from build123d import *

# Parameters (mm, degrees)
SKETCH1_R                   = 7.9375
BOSS_EXTRUDE1_DEPTH         = 9.525
SKETCH2_R                   = 4.7625
BOSS_EXTRUDE2_DEPTH         = 3.175
F_1_4_0_25_DIAMETER_HOLE1_D = 6.35
F_10_32_TAPPED_HOLE1_REACH  = 23.825
F_10_32_TAPPED_HOLE1_BORE_R = 2.0193


with BuildPart() as part:
    # Sketch1 → Boss-Extrude1 (new body)
    with BuildSketch(Plane(origin=(0, 0, 0), x_dir=(1, 0, 0), z_dir=(0, 1, 0))):
        with Locations(Location((0, 0, 0), (0, 0, 90))):
            Circle(SKETCH1_R)
    extrude(amount=BOSS_EXTRUDE1_DEPTH)

    # Sketch2 → Boss-Extrude2 (add)
    with BuildSketch(Plane(origin=(0, 9.525, 0), x_dir=(1, 0, 0), z_dir=(0, 1, 0))):
        with Locations(Location((0, 0, 0), (0, 0, 270))):
            Circle(SKETCH2_R)
    extrude(amount=BOSS_EXTRUDE2_DEPTH)

    # 1/4 (0.25) Diameter Hole1 (through all)
    with Locations(Plane(origin=(0, 0, 0), x_dir=(-1, 0, 0), z_dir=(0, -1, 0))):
        with Locations((0, 0)):
            Hole(F_1_4_0_25_DIAMETER_HOLE1_D / 2)

    # #10-32 Tapped Hole1 bore → #10-32 Tapped Hole1 (cut, up to next)
    with BuildSketch(Plane(origin=(0, 0, -7.9375), x_dir=(-1, 0, 0), z_dir=(0, 0, -1)), mode=Mode.PRIVATE) as f_10_32_tapped_hole1_sk1:
        with Locations((0, 4.7625)):
            Circle(F_10_32_TAPPED_HOLE1_BORE_R)
    f_10_32_tapped_hole1_tool1 = extrude(f_10_32_tapped_hole1_sk1.sketch, amount=-F_10_32_TAPPED_HOLE1_REACH, mode=Mode.PRIVATE) & part.part
    add(f_10_32_tapped_hole1_tool1.solids().sort_by_distance((0, 4.7625, -7.9375))[0], mode=Mode.SUBTRACT)


solid = part.part
The model under review builds one solid part; all positions refer to its coordinate system, in mm. A direction names the side the tool comes from. Coordinates: 2 decimals unless noted, no trailing zeros. Write each loop counter-clockwise with the first axis right and the second up, starting at its lowest first coordinate (ties: lowest second). Pieces come first, ordered by that corner, then holes. Notation, with made-up numbers: (82, -18) -> (122, -18) arc R7 cw to (122, -12) -> close; hole circle Ø5 at (18.5, 33). An arc over 180 degrees is marked (long way). Answer in a Markdown table with one row per item.
1. Draft analysis for pull direction X (two halves, no side actions). For faces 3 (the flat face through (3.4, 0, 0.1)), 4 (the cylindrical face through (-2.9, 11.09, -3.78)), 5 (the cylindrical face through (-0.93, 2.97, -5.23)), state which applies: +X half, -X half, draft (parallel to the pull), parting line (faces both ways), or undercut.
Answers below:
| item | result |
|---|---|
| face 3 | draft |
| face 4 | parting line |
| face 5 | undercut |
2. We need section D-D, the plane x = -2.25. State the section outline as (y, z) points (3 decimals), and give its area (3 significant figures).
Answers below:
| item | result |
|---|---|
| outline | (0, -7.612) -> (9.525, -7.612) -> (9.525, -4.197) -> (12.7, -4.197) -> (12.7, -2.24) -> (0, -2.24) -> close; (0, 2.24) -> (12.7, 2.24) -> (12.7, 4.197) -> (9.525, 4.197) -> (9.525, 7.612) -> (0, 7.612) -> close |
| area | 115 mm^2 |
3. For faces 1 (the flat face through (5, 9.525, 0)), 2 (the cylindrical face through (7.75, 4.7, 1.72)), list the 3-axis set-ups (+Z, -Z, +X, -X, +Y, -Y) from which the entire face can be reached by the end or side of a thin tool; tool diameter is ignored.
Answers below:
| item | result |
|---|---|
| face 1 | +Y |
| face 2 | +Y, -Y |
4. We need section B-B, the plane z = 0. State the section outline as (x, y) points (1 decimal), and give its area (3 significant figures).
Answers below:
| item | result |
|---|---|
| outline | (-7.9, 0) -> (-3.2, 0) -> (-3.2, 12.7) -> (-4.8, 12.7) -> (-4.8, 9.5) -> (-7.9, 9.5) -> close; (3.2, 0) -> (7.9, 0) -> (7.9, 9.5) -> (4.8, 9.5) -> (4.8, 12.7) -> (3.2, 12.7) -> close |
| area | 101 mm^2 |
5. Clearance check with flat-ended pins moving along their axes: pin 1 Ø2 at (x, y) = (2, 3.5) entering from -Z; pin 2 Ø5 at (x, y) = (-3, 11) entering from +Z; pin 3 Ø4 at (y, z) = (1.5, 6) entering from -X; pin 4 Ø5.5 at (x, z) = (0, 0) entering from -Y. State where each tip first meets the part, or that it passes through.
Answers below:
| item | result |
|---|---|
| pin 1 | stops at z = -7.86 |
| pin 2 | stops at z = 7.88 |
| pin 3 | stops at x = -6.86 |
| pin 4 | passes through |
6. Wall thickness on probe 1 along Y at (x, z) = (0, -4.6); probe 2 along Y at (x, z) = (-3, -6) (3 decimals); probe 3 along X at (y, z) = (2, -1.75): over which ranges is each line inside the solid? List them lowest first. Write a range as [from, to].
Answers below:
| item | result |
|---|---|
| probe 1 | y = [0, 2.74], [6.78, 12.7] |
| probe 2 | y = [0, 9.525] |
| probe 3 | x = [-7.74, -2.65], [2.65, 7.74] |
7. We need section A-A, the plane x = 0. State the section outline as (y, z) points (1 decimal), and give its area (3 significant figures).
Answers below:
| item | result |
|---|---|
| outline | (0, -7.9) -> (2.7, -7.9) -> (2.7, -3.2) -> (0, -3.2) -> close; (0, 3.2) -> (12.7, 3.2) -> (12.7, 4.8) -> (9.5, 4.8) -> (9.5, 7.9) -> (0, 7.9) -> close; (6.8, -7.9) -> (9.5, -7.9) -> (9.5, -4.8) -> (12.7, -4.8) -> (12.7, -3.2) -> (6.8, -3.2) -> close |
| area | 81.6 mm^2 |
